Geometry check sheet. Reference: the model listing, model coordinates, mm. Face numbers are marked on the shaded views. A direction names the side the tool comes from. Give positions to 0.01 mm unless a question says otherwise; leave off trailing zeros. Write each loop counter-clockwise with the first axis right and the second up, starting at its lowest first coordinate (ties: lowest second). Pieces come first, ordered by that corner, then holes. Notation, with made-up numbers: M 6.5,-11 L 31.5,-11 A7 ccw 31.5,-7 Z; hole C 69,6.25 d11. An arc over 180 degrees is marked long. One line per item, written item: value. Start each with the question number.
1. Tool access check on the marked faces 1 and 2. Record the directions out of +Z, -Z, +X, -X, +Y, -Y that give a thin tool (end or side, any length) a straight path to the whole face; none if there is none.
2. Gauge pin test, flat ends, axial feed: pin 1 (1 mm diameter, centred on x = 178, z = 297, fed in from -Y); pin 2 (1 mm diameter, centred on x = 532.5, y = -265, fed in from -Z); pin 3 (3 mm diameter, centred on x = 260, y = -96, fed in from +Z). Record the tip position at first contact, or that the pin passes through.
3. Scan line: line 1 (Z direction, x = 403.5, y = -227). Record every from-to range of solid material in increasing order.
4. Cross-section at B-B on z = 124.5. Record the cut outline in (x, y), then the cut area to 3 significant figures.
5. Cross-section at A-A on x = 646.5. Record the cut outline in (y, z), then the cut area to 3 significant figures.
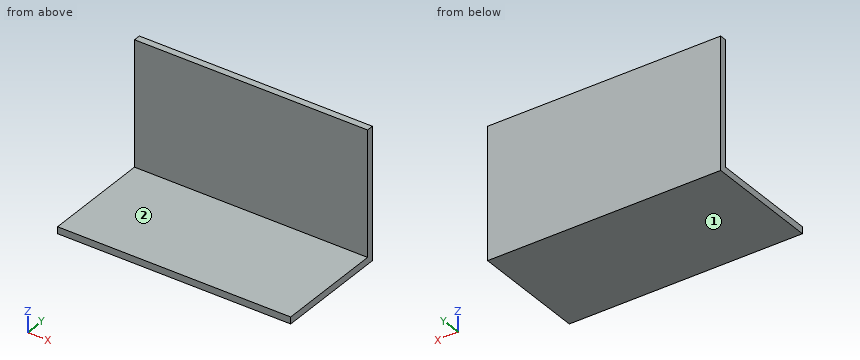
Autodesk Inventor part; units mm, degrees
ref_plane "plane_id6" through (0, -60, 0) normal (0, -1, 0) x (1, 0, 0)
ref_plane "YZ Plane" through (0, 0, 0) normal (1, 0, 0) x (0, 1, 0)
ref_plane "XZ Plane" through (0, 0, 0) normal (0, 1, 0) x (-1, 0, 0)
sketch "Skizze1" plane through (0, 0, 0) normal (0, 1, 0) x (-1, 0, 0)
  line L0 (0, 0) -> (-750, 0)
  line L1 (-750, 0) -> (-750, 422)
  line L2 (-750, 422) -> (0, 422)
  line L3 (0, 422) -> (0, 0)
  dimension "d0" = 750
  dimension "d1" = 422
extrude "Back_Back" add sketch "Skizze1" along normal blind 22
sketch "Skizze2" plane through (0, 0, 0) normal (0, -1, 0) x (1, 0, 0)
  line L0 (750, 422) -> (750, 0)
  line L1 (0, 0) -> (750, 0)
  line L2 (750, 0) -> (750, 22)
  line L3 (750, 22) -> (0, 22)
  line L4 (0, 22) -> (0, 0)
  dimension "d4" = 22
extrude "Back_Down" add sketch "Skizze2" along normal blind 350
sketch "Sketch_Footprint_Magnet&Robot" plane through (0, 0, 22) normal (0, 0, 1) x (1, 0, 0)
  line L0 (0, -350) -> (0, 22) construction
  line L1 (750, -350) -> (0, -350) construction
  line L2 (0, -200) -> (750, -200) construction
  line L3 (12, -45) -> (315, -45)
  line L4 (315, -45) -> (315, -355)
  line L5 (315, -355) -> (12, -355)
  line L6 (12, -355) -> (12, -45)
  line L7 (12, -45) -> (315, -355) construction
  line L8 (315, -45) -> (12, -355) construction
  line L9 (0, -100) -> (12, -100)
  line L10 (12, -100) -> (12, -300)
  line L11 (12, -300) -> (0, -300)
  line L12 (0, -300) -> (0, -100)
  line L13 (315, -100) -> (327, -100)
  line L14 (327, -100) -> (327, -300)
  line L15 (327, -300) -> (315, -300)
  line L16 (315, -300) -> (315, -100)
  line L17 (545, -265) -> (675, -265)
  line L18 (675, -265) -> (675, -135)
  line L19 (675, -135) -> (545, -135)
  line L20 (545, -135) -> (545, -265)
  line L21 (545, -265) -> (675, -135) construction
  line L22 (675, -265) -> (545, -135) construction
  line L23 (750, 0) -> (750, -350)
  line L24 (0, 0) -> (750, 0)
  point P0 (163.5, -200)
  point P1 (327, -200)
  point P2 (610, -200)
  dimension "d15" = 150
  dimension "d16" = 303
  dimension "d17" = 310
  dimension "d18" = 12
  dimension "d19" = 200
  dimension "d20" = 130
  dimension "d21" = 140
  dimension "d56" = 200
sketch "Sketch_ReferenceBoard" plane through (0, 0, 0) normal (0, -1, 0) x (1, 0, 0)
  line L0 (750, 422) -> (330, 422)
  line L1 (330, 422) -> (330, 125)
  line L2 (330, 125) -> (750, 125)
  line L3 (750, 125) -> (750, 422)
  line L4 (330, 446) -> (330, 125)
  line L5 (345, 330) -> (345, 130) construction
  line L6 (345, 130) -> (645, 130) construction
  line L7 (345, 208) -> (345, 130)
  line L8 (610, 22) -> (610, 130) construction
  line L9 (675, 22) -> (675, 130) construction
  line L10 (750, 422) -> (750, 22) construction
  line L11 (330, 360) -> (750, 360) construction
  line L12 (685, 422) -> (685, 125) construction
  line L13 (345, 400) -> (425, 400)
  line L14 (425, 400) -> (425, 320)
  line L15 (425, 320) -> (345, 320)
  line L16 (345, 320) -> (345, 400)
  line L17 (345, 400) -> (425, 320) construction
  line L18 (425, 400) -> (345, 320) construction
  line L19 (545, 400) -> (625, 400)
  line L20 (625, 400) -> (625, 320)
  line L21 (625, 320) -> (545, 320)
  line L22 (545, 320) -> (545, 400)
  line L23 (545, 400) -> (625, 320) construction
  line L24 (625, 400) -> (545, 320) construction
  line L25 (645, 220) -> (725, 220)
  line L26 (725, 220) -> (725, 300)
  line L27 (725, 300) -> (645, 300)
  line L28 (645, 300) -> (645, 220)
  line L29 (645, 220) -> (725, 300) construction
  line L30 (725, 220) -> (645, 300) construction
  line L31 (645, 130) -> (725, 130)
  line L32 (725, 130) -> (725, 210)
  line L33 (725, 210) -> (645, 210)
  line L34 (645, 210) -> (645, 130)
  line L35 (645, 130) -> (725, 210) construction
  line L36 (725, 130) -> (645, 210) construction
  line L37 (485, 303.4315) -> (541.5685, 360)
  line L38 (541.5685, 360) -> (485, 416.5685)
  line L39 (485, 416.5685) -> (428.4315, 360)
  line L40 (428.4315, 360) -> (485, 303.4315)
  line L41 (485, 303.4315) -> (485, 416.5685) construction
  line L42 (541.5685, 360) -> (428.4315, 360) construction
  line L43 (685, 303.4315) -> (741.5685, 360)
  line L44 (741.5685, 360) -> (685, 416.5685)
  line L45 (685, 416.5685) -> (628.4315, 360)
  line L46 (628.4315, 360) -> (685, 303.4315)
  line L47 (685, 303.4315) -> (685, 416.5685) construction
  line L48 (741.5685, 360) -> (628.4315, 360) construction
  point P0 (0, 0)
  point P1 (163.5, 22)
  point P2 (685, 360)
  point P3 (585, 360)
  point P4 (485, 360)
  point P5 (385, 360)
  point P6 (685, 260)
  point P7 (685, 170)
  dimension "d7" = 297
  dimension "d8" = 420
  dimension "d24" = 330
  dimension "d25" = 75
  dimension "d26" = 108
  dimension "d28" = 55
  dimension "d29" = 100
  dimension "d30" = 100
  dimension "d31" = 100
  dimension "d32" = 235
  dimension "d33" = 100
  dimension "d34" = 90
  dimension "d35" = 80
  dimension "d36" = 80
  dimension "d37" = 45
ref_plane "plane_id6" through (0, -60, 0) normal (0, -1, 0) x (1, 0, 0)
sketch "Sketch_RefrenceBoard_id6" plane through (0, -60, 0) normal (0, -1, 0) x (1, 0, 0)
  line L0 (405, 138.5685) -> (461.5685, 82)
  line L1 (461.5685, 82) -> (405, 25.4315)
  line L2 (405, 25.4315) -> (348.4315, 82)
  line L3 (348.4315, 82) -> (405, 138.5685)
  line L4 (0, 22) -> (750, 22) construction
  line L5 (405, 138.5685) -> (405, 25.4315) construction
  line L6 (348.4315, 82) -> (461.5685, 82) construction
  point P0 (0, 0)
  point P1 (405, 82)
  point P2 (345, 130)
  point P3 (405, 82)
  dimension "d40" = 45
  dimension "d41" = 80
  dimension "d42" = 60
  dimension "d43" = 60
  dimension "d45" = 3.4315
  dimension "d46" = 3.4315
sketch "Sketch_Magnet_Back" plane through (0, 0, 0) normal (0, -1, 0) x (1, 0, 0)
  line L0 (318, 369.7147) -> (318, 209.7147)
  line L1 (12, 209.7147) -> (12, 369.7147)
  line L2 (12, 363) -> (318, 363)
  line L3 (318, 363) -> (318, 53)
  line L4 (318, 53) -> (12, 53)
  line L5 (12, 53) -> (12, 363)
  line L6 (12, 121.0397) -> (0, 121.0397)
  line L7 (0, 121.0397) -> (0, 22)
  line L8 (0, 22) -> (12, 22)
  line L9 (12, 22) -> (12, 121.0397)
  line L10 (318, 121.0397) -> (330, 121.0397)
  line L11 (330, 121.0397) -> (330, 22)
  line L12 (330, 22) -> (318, 22)
  line L13 (318, 22) -> (318, 121.0397)
  line L14 (750, 22) -> (0, 22) construction
  line L15 (0, 22) -> (0, 0) construction
  line L16 (12, 128) -> (318, 128) construction
  line L17 (318, 128) -> (318, 288) construction
  line L18 (318, 288) -> (12, 288) construction
  line L19 (12, 288) -> (12, 128) construction
  line L20 (12, 128) -> (318, 288) construction
  line L21 (318, 128) -> (12, 288) construction
  point P0 (318, 208)
  point P1 (165, 208)
  point P2 (12, 208)
  point P3 (12, 208)
  point P4 (165, 128)
  point P5 (165, 288)
  point P6 (345, 130)
  dimension "d47" = 306
  dimension "d48" = 12
  dimension "d51" = 186
  dimension "d52" = 310
  dimension "d53" = 160
  dimension "d54" = 180
  dimension "d55" = 78
properties part number "Referenzboard"
Report:
1. face 1: -Z, +X, -X, +Y, -Y
1. face 2: +Z, +X, -X, -Y
2. pin 1: stops at y = 0
2. pin 2: stops at z = 0
2. pin 3: stops at z = 22
3. line 1: z = 0 to 22
4. outline: M 0,0 L 750,0 L 750,22 L 0,22 Z
4. area: 16,500 mm^2
5. outline: M -350,0 L 22,0 L 22,422 L 0,422 L 0,22 L -350,22 Z
5. area: 17,000 mm^2
